Check sheet for the modelled part. Datum: model origin and axes. Units: mm. Face numbers are marked on the shaded views. Give positions to 0.01 mm unless a question says otherwise; leave off trailing zeros. Write each loop counter-clockwise with the first axis right and the second up, starting at its lowest first coordinate (ties: lowest second). Pieces come first, ordered by that corner, then holes. Notation, with made-up numbers: M 36,77 L 47,77 A19 cw 47,106 Z; hole C 58,26 d2. An arc over 180 degrees is marked long. Write item = value, one per line. Start each with the question number.
1) Mould release check, pull along Z, two halves, no side actions. Record for the marked faces 1, 2 and 3: released by +Z, released by -Z, zero draft, split by the parting line, or undercut.
2) Cross-section at D-D, the plane y = 19.5. Record the cut outline in (x, z).
3) Cross-section at A-A, the plane y = 4. Record the cut outline in (x, z), plus the area to 3 significant figures.
4) Cross-section at B-B, the plane z = -0.5. Record the cut outline in (x, y).
5) Scan lines: line 1 along Y through (x, z) = (0.05, -0.5); line 2 along Z through (x, y) = (0.65, 3.25); line 3 along Y through (x, z) = (0.75, 0). Record each from-to range of solid material in increasing order. Write a range as [from, to].
Autodesk Inventor part; units mm, degrees
ref_plane "YZ Plane" through (0, 0, 0) normal (1, 0, 0) x (0, 1, 0)
ref_plane "XZ Plane" through (0, 0, 0) normal (0, 1, 0) x (-1, 0, 0)
ref_plane "XY Plane" through (0, 0, 0) normal (0, 0, 1) x (1, 0, 0)
sketch "Sketch1" plane through (0, 0, 0) normal (0, 1, 0) x (-1, 0, 0)
  line L0 (-1.3, -3.75) -> (1.3, -3.75)
  line L1 (1.3, -3.75) -> (1.3, 3.75)
  line L2 (1.3, 3.75) -> (-1.3, 3.75)
  line L3 (-1.3, 3.75) -> (-1.3, -3.75)
  line L4 (-1.3, -3.75) -> (1.3, 3.75) construction
  line L5 (1.3, -3.75) -> (-1.3, 3.75) construction
  point P0 (0, 0)
  dimension "d0" = 2.6
  dimension "d1" = 7.5
extrude "Extrusion1" add sketch "Sketch1" along normal blind 25
chamfer "Chamfer1" distance 7.5 angle 45 1 edges at (0, 25, -3.75)
sketch "Sketch2" plane through (1.3, 0, 3.75) normal (1, 0, 0) x (0, 0, -1)
  circle A0 centre (3.75, 4) radius 1.5
  point P0 (3.75, 0)
  dimension "d7" = 3
  dimension "d8" = 4
extrude "Extrusion2" cut sketch "Sketch2" against normal blind 16
properties part number "locker"
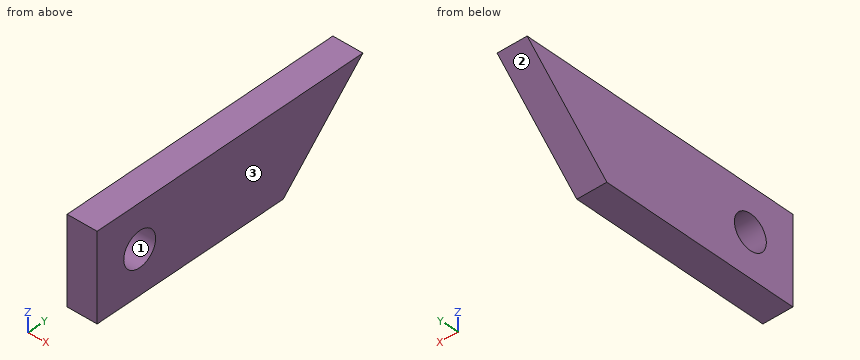
Reply:
q1.face_1 = undercut
q1.face_2 = released by -Z
q1.face_3 = zero draft
q2.outline = M -1.3,-1.75 L 1.3,-1.75 L 1.3,3.75 L -1.3,3.75 Z
q3.outline = M -1.3,-3.75 L 1.3,-3.75 L 1.3,-1.5 L -1.3,-1.5 Z; M -1.3,1.5 L 1.3,1.5 L 1.3,3.75 L -1.3,3.75 Z
q3.area = 11.7 mm2
q4.outline = M -1.3,0 L 1.3,0 L 1.3,2.59 L -1.3,2.59 Z; M -1.3,5.41 L 1.3,5.41 L 1.3,20.75 L -1.3,20.75 Z
q5.line_1 = [0, 2.59], [5.41, 20.75]
q5.line_2 = [-3.75, -1.3], [1.3, 3.75]
q5.line_3 = [0, 2.5], [5.5, 21.25]
